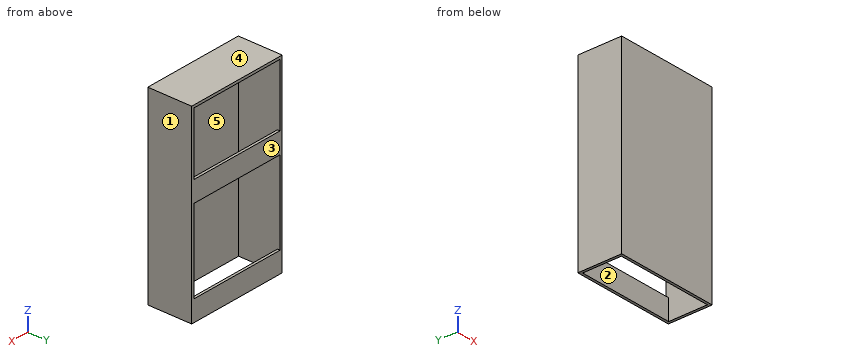
Autodesk Inventor part; units mm, degrees
ref_plane "YZ Plane" through (0, 0, 0) normal (1, 0, 0) x (0, 1, 0)
ref_plane "XZ Plane" through (0, 0, 0) normal (0, 1, 0) x (-1, 0, 0)
ref_plane "XY Plane" through (0, 0, 0) normal (0, 0, 1) x (1, 0, 0)
sketch "Sketch1" plane through (0, 0, 0) normal (0, 1, 0) x (-1, 0, 0)
  line L0 (0, 0) -> (-127, 0)
  line L1 (-127, 0) -> (-127, 228.6)
  line L2 (-127, 228.6) -> (0, 228.6)
  line L3 (0, 228.6) -> (0, 0)
  dimension "d0" = 127
  dimension "d1" = 228.6
extrude "Extrusion1" add sketch "Sketch1" along normal blind 3.175
sketch "Sketch2" plane through (0, 3.175, 0) normal (0, 1, 0) x (1, 0, 0)
  line L0 (0, 0) -> (0, -228.6)
  line L1 (0, 0) -> (3.175, 0)
  line L2 (3.175, 0) -> (3.175, -228.6)
  line L3 (3.175, -228.6) -> (0, -228.6)
  line L4 (0, -228.6) -> (0, 0)
  dimension "d4" = 3.175
  dimension "d5" = 228.6
extrude "Extrusion2" add sketch "Sketch2" along normal blind 50.8
sketch "Sketch3" plane through (0, 3.175, 0) normal (0, 1, 0) x (1, 0, 0)
  line L0 (127, -228.6) -> (127, 0)
  line L1 (127, 0) -> (123.825, 0)
  line L2 (123.825, 0) -> (123.825, -228.6)
  line L3 (123.825, -228.6) -> (127, -228.6)
  line L4 (127, -228.6) -> (127, 0)
  point P0 (0, 0)
  dimension "d8" = 3.175
  dimension "d9" = 228.6
extrude "Extrusion3" add sketch "Sketch3" along normal blind 50.8
sketch "Sketch6" plane through (0, 0, 228.6) normal (0, 0, 1) x (1, 0, 0)
  line L0 (0, 0) -> (127, 0)
  line L1 (0, 53.975) -> (127, 53.975)
  line L2 (127, 53.975) -> (127, 0)
  line L3 (127, 0) -> (0, 0)
  line L4 (0, 0) -> (0, 53.975)
extrude "Extrusion4" add sketch "Sketch6" along normal blind 3.175
sketch "Sketch7" plane through (3.175, 3.175, 0) normal (1, 0, 0) x (0, 0, -1)
  line L0 (-228.6, 50.8) -> (-152.4, 50.8) construction
  line L1 (0, 50.8) -> (-231.775, 50.8) construction
  line L2 (-228.6, 50.8) -> (-152.4, 50.8) construction
  line L3 (-152.4, 50.8) -> (-127, 50.8)
  line L4 (-127, 50.8) -> (-127, 47.625)
  line L5 (-127, 47.625) -> (-152.4, 47.625)
  line L6 (-152.4, 47.625) -> (-152.4, 50.8)
  point P0 (0, -3.175)
  dimension "d19" = 76.2
  dimension "d20" = 0
  dimension "d21" = 25.4
  dimension "d22" = 3.175
extrude "Extrusion5" add sketch "Sketch7" along normal blind 120.65
sketch "Sketch8" plane through (0, 53.975, 0) normal (0, 1, 0) x (1, 0, 0)
  line L0 (3.175, -127) -> (3.175, 0)
  line L1 (3.175, 0) -> (123.825, 0)
  line L2 (123.825, 0) -> (123.825, -25.4)
  line L3 (123.825, -25.4) -> (3.175, -25.4)
  line L4 (3.175, -25.4) -> (3.175, 0)
  point P0 (0, 0)
  point P1 (3.175, -25.4)
  dimension "d25" = 120.65
  dimension "d26" = 25.4
extrude "Extrusion6" add sketch "Sketch8" against normal blind 3.175
properties part number "ShootingMech_Housing"
Verification items for the finished model (mm, model axes). Face numbers are marked on the shaded views. A direction names the side the tool comes from. Coordinates: 2 decimals unless noted, no trailing zeros. Order: outer loops, then holes, each group sorted by start corner. A loop starts at its lowest first (then second) coordinate and runs counter-clockwise, first axis right, second up. Notation, with made-up numbers: M 45.5,29.25 L 72.5,29.25 A21 cw 72.5,58.25 Z; hole C 76.25,-6.5 d5. An arc over 180 degrees is marked long. One line per item, written item: value. Start each with the question number.
Item 1: Depth check by flat-ended pin: P1, Ø5, axis at x = 22.5, z = 180, coming from the +Y side (3 decimals); P2, Ø4, axis at x = 53.5, y = 16, coming from the -Z side. Enter the tip coordinate at first touch or a pass-through.
Item 2: Sectioned sample at C-C on z = 49.5. Record the cut outline in (x, y) (3 decimals).
Item 3: Sectioned sample at B-B on z = 143.5. Record the cut outline in (x, y) (3 decimals).
Item 4: Access from +Z, -Z, +X, -X, +Y, -Y to the whole of each face (thin tool, end or side, straight path). Record for the marked faces 4 and 5.
Item 5: Sectioned sample at A-A on x = 17. Record the cut outline in (y, z) (3 decimals), then the cut area to 3 significant figures.
Item 6: Thickness scan on probe 1 along X at (y, z) = (14, 146.5) (3 decimals); probe 2 along Y at (x, z) = (61.5, 127.5) (3 decimals); probe 3 along Z at (x, y) = (70, 49) (3 decimals). Record the ranges inside material, lowest first.
Item 7: Sectioned sample at D-D on y = 24.5. Record the cut outline in (x, z) (3 decimals).
Item 8: Mould release check, pull along Y, two halves, no side actions. Record for the marked faces 1, 2 and 3: pulls with the +Y half, pulls with the -Y half, needs draft (parallel to the pull), parting line crosses it, or undercut.
Calculated:
1. P1: y = 3.175
1. P2: z = 228.6
2. outline: M 0,0 L 127,0 L 127,53.975 L 123.825,53.975 L 123.825,3.175 L 3.175,3.175 L 3.175,53.975 L 0,53.975 Z
3. outline: M 0,0 L 127,0 L 127,53.975 L 0,53.975 Z; hole M 3.175,3.175 L 123.825,3.175 L 123.825,50.8 L 3.175,50.8 Z
4. face 4: +Z, +X, -X, +Y, -Y
4. face 5: -Z
5. outline: M 0,0 L 3.175,0 L 3.175,228.6 L 53.975,228.6 L 53.975,231.775 L 0,231.775 Z; M 50.8,0 L 53.975,0 L 53.975,25.4 L 50.8,25.4 Z; M 50.8,127 L 53.975,127 L 53.975,152.4 L 50.8,152.4 Z
5. area: 1,060 mm^2
6. probe 1: 0 to 3.175, 123.825 to 127
6. probe 2: 0 to 3.175, 50.8 to 53.975
6. probe 3: 228.6 to 231.775
7. outline: M 0,0 L 3.175,0 L 3.175,228.6 L 123.825,228.6 L 123.825,0 L 127,0 L 127,231.775 L 0,231.775 Z
8. face 1: needs draft
8. face 2: undercut
8. face 3: pulls with the +Y half
